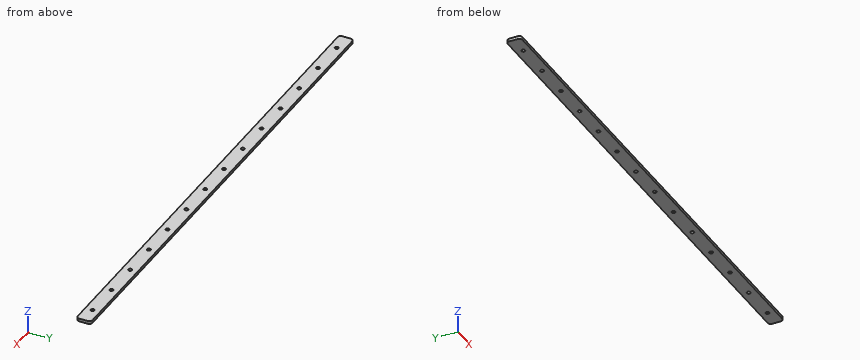
Autodesk Inventor part; units mm, degrees
ref_plane "YZ Plane" through (0, 0, 0) normal (1, 0, 0) x (0, 1, 0)
ref_plane "XZ Plane" through (0, 0, 0) normal (0, 1, 0) x (-1, 0, 0)
ref_plane "XY Plane" through (0, 0, 0) normal (0, 0, 1) x (1, 0, 0)
sketch "Sketch1" plane through (0, 0, 0) normal (0, 0, 1) x (1, 0, 0)
  line L0 (0, 0) -> (350, 0)
  line L1 (350, 0) -> (350, 10)
  line L2 (350, 10) -> (0, 10)
  line L3 (0, 10) -> (0, 0)
  dimension "d0" = 350
  dimension "d1" = 10
extrude "Extrusion1" add sketch "Sketch1" along normal blind 2
sketch "Sketch2" plane through (0, 0, 2) normal (0, 0, 1) x (1, 0, 0)
  line L0 (0, 10) -> (0, 0)
  point P0 (13, 5)
  point P1 (0, 5)
  dimension "d4" = 13
hole "Hole1" at (13, 5, 2) direction (0, 0, -1) diameter 2.459 end through all
pattern_linear "Rectangular Pattern1" count 14 spacing 25 along (1, 0, 0) of "Hole1"
fillet "Fillet1" radius 2 4 edges at (0, 0, 1) (0, 10, 1) (350, 0, 1) (350, 10, 1)
properties part number "Linear Rail Screw Plate"
Part model, mm, in its own coordinate system. Give positions to 0.01 mm unless a question says otherwise; leave off trailing zeros. Use one line per item in the form item = value.
Item 1: Probe probe 1 along Y at (x, z) = (188, 1.1). List the from-to ranges inside material, lowest first. Write a range as from..to.
Solution:
probe_1 = 0..3.77, 6.23..10
Item 2: Slice it at A-A on z = 1.2. Count the separate pieces of the cut face and the enclosed holes in it, and give its area (3 significant figures).
Solution:
separate_pieces = 1
enclosed_holes = 14
area = 3,430 mm2
Item 3: Pin check, flat tip, straight feed: pin 1 Ø2 at (x, y) = (13, 5) entering from -Z. Stop position of the tip, or through.
Solution:
pin_1 = through
